The model under review builds one solid part; all positions refer to its coordinate system, in mm. Face numbers are marked on the shaded views. A direction names the side the tool comes from. Round coordinates to 2 decimals unless told otherwise and drop trailing zeros. Write each loop counter-clockwise with the first axis right and the second up, starting at its lowest first coordinate (ties: lowest second). Pieces come first, ordered by that corner, then holes.
Item 1: Add section B-B (y = -3.5). Give the boundary of the cut face in (x, z), plus the area to 3 significant figures.
Item 2: Add section C-C (x = 9). Give the boundary of the cut face in (y, z).
Item 3: Draft analysis for pull direction X (two halves, no side actions). For the marked faces 4, 5, 6 and 7, state which applies: +X half, -X half, draft (parallel to the pull), parting line (faces both ways), or undercut.
Item 4: Add section A-A (y = -24.5). Give the boundary of the cut face in (x, z).
Item 5: Add section D-D (z = 6.5). Give the boundary of the cut face in (x, y), plus the area to 3 significant figures.
Item 6: To check wall thickness, follow L1, parallel to Z at x = 0, y = -2; L2, parallel to X at y = -3, z = 8; L3, parallel to Y at x = 4.75, z = 0.25. State the ranges of each line that lie inside material, in increasing order.
Item 7: Clearance check with flat-ended pins moving along their axes: pin 1 Ø3 at (x, z) = (6.5, -0.5) entering from -Y; pin 2 Ø4 at (x, z) = (9.76, -3.52) entering from +Y; pin 3 Ø1.4 at (x, z) = (5.5, 8) entering from +Y. State where each tip first meets the part, or that it passes through.
Item 8: Machinability: for the marked faces 1, 2 and 3, which of the approach directions +Z, -Z, +X, -X, +Y, -Y give a long, thin tool a straight path to every point of the face, cutting with its end or side? Answer none if there is none.
Autodesk Inventor part; units mm, degrees
ref_plane "YZ Plane" through (0, 0, 0) normal (1, 0, 0) x (0, 1, 0)
ref_plane "XZ Plane" through (0, 0, 0) normal (0, 1, 0) x (-1, 0, 0)
ref_plane "XY Plane" through (0, 0, 0) normal (0, 0, 1) x (1, 0, 0)
sketch "Sketch1" plane through (0, 0, 0) normal (0, 1, 0) x (-1, 0, 0)
  circle A0 centre (-0.062958, 8.481909) radius 2.4
  circle A1 centre (-0.362958, -3.518091) radius 2.15
  circle A2 centre (-10.062958, 8.481909) radius 2.4
  circle A3 centre (-9.762958, -3.518091) radius 2.15
  point P0 (0, 0)
  dimension "d0" = 4.8
  dimension "d1" = 4.3
  dimension "d3" = 4.8
  dimension "d5" = 4.3
  dimension "d24" = 10
  dimension "d25" = 0.3
  dimension "d26" = 0.3
extrude "Extrusion1" add sketch "Sketch1" along normal blind 6 contours A0 | A2
sketch "Sketch2" plane through (0.062958, 0, 8.481909) normal (0, -1, 0) x (1, 0, 0)
  circle A0 centre (0.3, -12) radius 2.15
  circle A1 centre (9.7, -12) radius 2.15
  circle A2 centre (10, 0) radius 2.4
  circle A3 centre (0, 0) radius 2.4
  line L0 (-2.4, 0) -> (-1.85, -12)
  line L1 (0.3, -14.15) -> (9.7, -14.15)
  line L2 (11.85, -12) -> (12.39746, -0.110392)
  line L3 (0, 2.4) -> (10, 2.4)
  point P0 (-0.062958, -8.481909)
sketch "Sketch3" plane through (0.062958, 0, 8.481909) normal (0, -1, 0) x (1, 0, 0)
  circle A0 centre (10, 0) radius 2.4
  circle A1 centre (0, 0) radius 2.4
  line L0 (0, -2.4) -> (10, -2.4)
  line L1 (0, -2.4) -> (10, -2.4)
  circle A2 centre (0, 0) radius 2.4
  circle A3 centre (10, 0) radius 2.4
  circle A4 centre (10, 0) radius 2.4
  circle A5 centre (0, 0) radius 2.4
  circle A6 centre (0, 0) radius 2.4
  circle A7 centre (0, 0) radius 2.4
  circle A8 centre (0, 0) radius 2.4
  circle A9 centre (10, 0) radius 2.4
  circle A10 centre (10, 0) radius 2.4
  circle A11 centre (10, 0) radius 2.4
  circle A12 centre (10, 0) radius 2.4
  circle A13 centre (0, 0) radius 2.4
  circle A14 centre (10, 0) radius 2.4
  circle A15 centre (10, 0) radius 2.4
  circle A16 centre (0, 0) radius 2.4
  line L2 (0, 2.4) -> (10, 2.4)
  point P0 (-0.062958, -8.481909)
  point P1 (-2.4, 0)
  point P2 (12.39746, -0.110392)
extrude "Extrusion2" add sketch "Sketch3" along normal blind 18
sketch "Sketch4" plane through (0.062958, -18, 8.481909) normal (0, -1, 0) x (1, 0, 0)
  circle A0 centre (0.3, -12) radius 2.15
  circle A1 centre (9.7, -12) radius 2.15
  circle A2 centre (0, 0) radius 2.4
  circle A3 centre (10, 0) radius 2.4
  arc A4 (0, -2.4) -> (0, 2.4) centre (0, 0) ccw
  arc A5 (10, 2.4) -> (10, -2.4) centre (10, 0) ccw
  arc A6 (0, 2.4) -> (0, -2.4) centre (0, 0) ccw
  arc A7 (10, -2.4) -> (10, 2.4) centre (10, 0) ccw
  line L0 (0, -2.4) -> (10, -2.4)
  line L1 (0, -2.4) -> (10, -2.4)
  line L2 (10, 2.4) -> (0, 2.4)
  line L3 (10, 2.4) -> (0, 2.4)
  circle A8 centre (0, 0) radius 2.4
  arc A9 (0, -2.4) -> (0, 2.4) centre (0, 0) ccw
  arc A10 (0, 2.4) -> (0, -2.4) centre (0, 0) ccw
  circle A11 centre (10, 0) radius 2.4
  arc A12 (10, 2.4) -> (10, -2.4) centre (10, 0) ccw
  arc A13 (10, -2.4) -> (10, 2.4) centre (10, 0) ccw
  arc A14 (10, 2.4) -> (10, -2.4) centre (10, 0) ccw
  line L4 (0, -2.4) -> (10, -2.4)
  arc A15 (0, -2.4) -> (0, 2.4) centre (0, 0) ccw
  line L5 (10, 2.4) -> (0, 2.4)
  line L6 (0, -2.4) -> (10, -2.4)
  arc A16 (10, -2.4) -> (10, 2.4) centre (10, 0) ccw
  line L7 (10, 2.4) -> (0, 2.4)
  arc A17 (0, 2.4) -> (0, -2.4) centre (0, 0) ccw
  line L8 (0, -2.4) -> (10, -2.4)
  line L9 (0, -2.4) -> (10, -2.4)
  line L10 (10, 2.4) -> (0, 2.4)
  line L11 (10, 2.4) -> (0, 2.4)
  circle A18 centre (0, 0) radius 2.4
  circle A19 centre (10, 0) radius 2.4
  circle A20 centre (0, 0) radius 2.4
  circle A21 centre (10, 0) radius 2.4
  circle A22 centre (0.3, -12) radius 2.15
  circle A23 centre (9.7, -12) radius 2.15
  circle A24 centre (10, 0) radius 2.4
  circle A25 centre (0, 0) radius 2.4
  line L12 (-2.4, 0) -> (-1.85, -12)
  line L13 (0.3, -14.15) -> (9.7, -14.15)
  line L14 (11.85, -12) -> (12.39746, -0.110392)
  line L15 (0, 2.4) -> (10, 2.4)
  point P0 (-0.062958, -8.481909)
  point P1 (-0.062958, -8.481909)
  point P2 (-0.062958, -8.481909)
sketch "Sketch4 outline for Extrusion3" plane through (0.062958, -18, 8.481909) normal (0, -1, 0) x (1, 0, 0)
  line L0 (-2.4, 0) -> (-1.85, -12)
  arc A0 (0, 2.4) -> (-2.4, 0) centre (0, 0) ccw
  line L1 (10, 2.4) -> (0, 2.4)
  arc A1 (12.39746, -0.110392) -> (10, 2.4) centre (10, 0) ccw
  line L2 (11.85, -12) -> (12.39746, -0.110392)
  arc A2 (9.7, -14.15) -> (11.85, -12) centre (9.7, -12) ccw
  line L3 (0.3, -14.15) -> (9.7, -14.15)
  arc A3 (-1.85, -12) -> (0.3, -14.15) centre (0.3, -12) ccw
extrude "Extrusion3" add sketch "Sketch4 outline for Extrusion3" along normal blind 4
sketch "Sketch5" plane through (0.062958, -22, 8.481909) normal (0, -1, 0) x (1, 0, 0)
  arc A0 (-1.85, -12) -> (0.3, -14.15) centre (0.3, -12) ccw
  circle A1 centre (0.3, -12) radius 2.15
  arc A2 (9.7, -14.15) -> (11.85, -12) centre (9.7, -12) ccw
  circle A3 centre (9.7, -12) radius 2.15
  point P0 (-0.062958, -8.481909)
  point P1 (0.3, -14.15)
extrude "Extrusion4" add sketch "Sketch5" along normal blind 3.5
sketch "Sketch6" plane through (0.362958, -25.5, -3.518091) normal (0, -1, 0) x (1, 0, 0)
  arc A0 (0, -2.15) -> (-2.15, 0) centre (0, 0) ccw
  circle A1 centre (0, 0) radius 2
  arc A2 (11.55, 0) -> (9.4, -2.15) centre (9.4, 0) ccw
  circle A3 centre (9.4, 0) radius 2
  point P0 (-0.362958, 3.518091)
  dimension "d15" = 4
  dimension "d16" = 4
extrude "Extrusion5" add sketch "Sketch6" along normal blind 2
sketch "Sketch7" plane through (0.362958, -27.5, -3.518091) normal (0, -1, 0) x (1, 0, 0)
  circle A0 centre (0, 0) radius 1.5
  circle A1 centre (9.4, 0) radius 2
  circle A2 centre (9.4, 0) radius 1.5
  point P0 (-0.362958, 3.518091)
  dimension "d19" = 3
  dimension "d20" = 3
extrude "Extrusion6" cut sketch "Sketch7" against normal blind 6 contours A0 | A2
sketch "Sketch8" plane through (0.062958, 6, 8.481909) normal (0, 1, 0) x (1, 0, 0)
  circle A0 centre (0, 0) radius 1.5
  circle A1 centre (10, 0) radius 2.4
  circle A2 centre (10, 0) radius 1.5
  point P0 (-0.062958, 8.481909)
  dimension "d27" = 3
  dimension "d28" = 3
extrude "Extrusion7" cut sketch "Sketch8" against normal blind 10 contours A0 | A2
properties part number "gripper3rightsideservoholder_3DPrint"
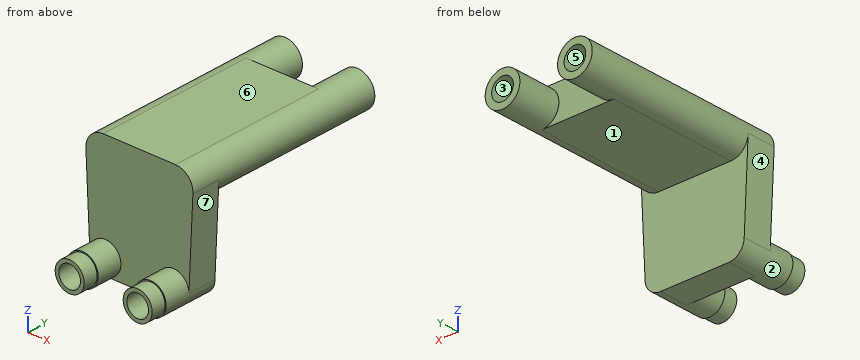
Numbers:
1. outline: (0.06, 6.08) - (10.06, 6.08) arc R2.4 ccw to (10.06, 10.88) - (0.06, 10.88) arc R2.4 ccw to start; hole circle Ø3 at (0.06, 8.48); hole circle Ø3 at (10.06, 8.48)
1. area: 52.0 mm2
2. outline: (-27.5, -5.37) - (-25.5, -5.37) - (-25.5, -5.53) - (-22, -5.53) - (-22, -5.67) - (-18, -5.67) - (-18, 6.08) - (0, 6.08) - (0, 6.33) - (6, 6.33) - (6, 7.42) - (-4, 7.42) - (-4, 9.54) - (6, 9.54) - (6, 10.63) - (0, 10.63) - (0, 10.88) - (-22, 10.88) - (-22, -1.51) - (-25.5, -1.51) - (-25.5, -1.67) - (-27.5, -1.67) - (-27.5, -2.23) - (-21.5, -2.23) - (-21.5, -4.81) - (-27.5, -4.81) - close
3. face 4: -X half
3. face 5: undercut
3. face 6: draft
3. face 7: +X half
4. outline: circle Ø4.3 at (0.36, -3.52); circle Ø4.3 at (9.76, -3.52); hole circle Ø3 at (0.36, -3.52); hole circle Ø3 at (9.76, -3.52)
5. outline: (-2.25, -22) - (12.37, -22) - (12.37, -18) - (11.42, -18) - (11.42, 6) - (8.71, 6) - (8.71, 0) - (1.42, 0) - (1.42, 6) - (-1.29, 6) - (-1.29, -18) - (-2.25, -18) - close
5. area: 320 mm2
6. L1: z = 6.08 to 6.98, 9.98 to 10.88
6. L2: x = -2.29 to -1.36, 1.48 to 8.64, 11.48 to 12.41
6. L3: y = -22 to -18
7. pin 1: stops at y = -22
7. pin 2: stops at y = -18
7. pin 3: stops at y = 0
8. face 1: -Z, +X, -X, +Y
8. face 2: -Y
8. face 3: +Y
